Design review of the part built by this model. Coordinates are the model's own, in mm. A direction names the side the tool comes from. Give positions to 0.01 mm unless a question says otherwise; leave off trailing zeros. Loops run counter-clockwise (first coordinate to the right, second up) from the corner with the lowest first, then second, coordinate; pieces in that order, holes last. Notation, with made-up numbers: (-26, 86) - (28, 86) arc R24 cw to (28, 111) - close; hole circle Ø2 at (7, 18.25). An arc over 180 degrees is marked (long way). Put each result on its own line as item: value. Start each with the question number.
```python
from build123d import *

# Parameters (mm, degrees)
F1_DEPTH = 314.325
F2_R     = 3.175
F3_DEPTH = 50.801
F4_R     = 3.175
F5_DEPTH = 50.801


with BuildPart() as f1:
    # F0 (on Right) → F1 (new body, symmetric)
    with BuildSketch(Plane.YZ):
        Polygon((0, 44.45), (0, 0), (6.35, 0), (6.35, 50.8), (-44.45, 50.8), (-44.45, 44.45), align=None)
    extrude(amount=F1_DEPTH, both=True)

    # F2 (on face) → F3 (cut, through all)
    with BuildSketch(Plane.XY.offset(50.8)):
        with Locations((-298.45, -19.05)):
            Circle(F2_R)
        with Locations((-105.56875, -19.05)):
            Circle(F2_R)
        with Locations((298.45, -19.05)):
            Circle(F2_R)
        with Locations((-148.43125, -19.05)):
            Circle(F2_R)
        with Locations((-21.43125, -19.05)):
            Circle(F2_R)
        with Locations((21.43125, -19.05)):
            Circle(F2_R)
        with Locations((105.56875, -19.05)):
            Circle(F2_R)
        with Locations((148.43125, -19.05)):
            Circle(F2_R)
    extrude(amount=-F3_DEPTH, mode=Mode.SUBTRACT)

    # F4 (on face) → F5 (cut, through all)
    with BuildSketch(Plane.XY.offset(50.8)):
        with Locations((-185.166, -19.05)):
            Circle(F4_R)
        with Locations((-61.722, -19.05)):
            Circle(F4_R)
        with Locations((61.722, -19.05)):
            Circle(F4_R)
        with Locations((185.166, -19.05)):
            Circle(F4_R)
    extrude(amount=-F5_DEPTH, mode=Mode.SUBTRACT)


solid = f1.part
```
Item 1: Consider section B-B (x = -123). State the section outline as (y, z) points, plus the area to 3 significant figures.
Item 2: For L1, parallel to Y at x = 272, z = 24; L2, parallel to Z at x = 264, y = -40.5; L3, parallel to Y at x = 298.45, z = 47.25 (3 decimals), list the stretches that pass through material, from the lowest coordinate up. Write a range as from..to.
Item 3: Consider section A-A (y = -36.5). State the section outline as (x, z) points (3 decimals), plus the area to 3 significant figures.
Item 4: Consider section C-C (z = 29.5). State the section outline as (x, y) points (3 decimals).
Item 5: For P1, Ø5.5, axis at x = 148.43, y = -19.05, coming from the -Z side; P2, Ø7.5, axis at x = -21.43, y = -19.05, coming from the -Z side, all flat-tipped, find the tip position at first contact; note any pin that passes through.
Item 6: Machinability: for faces 1 (the flat face through (4, -19, 50.8)), 2 (the flat face through (4, 0, 23)), which of the approach directions +Z, -Z, +X, -X, +Y, -Y give a long, thin tool a straight path to every point of the face, cutting with its end or side? Answer none if there is none.
Geometry says:
1. outline: (-44.45, 44.45) - (0, 44.45) - (0, 0) - (6.35, 0) - (6.35, 50.8) - (-44.45, 50.8) - close
1. area: 605 mm2
2. L1: y = 0..6.35
2. L2: z = 44.45..50.8
2. L3: y = -44.45..-22.225, -15.875..6.35
3. outline: (-314.325, 44.45) - (314.325, 44.45) - (314.325, 50.8) - (-314.325, 50.8) - close
3. area: 3,990 mm2
4. outline: (-314.325, 0) - (314.325, 0) - (314.325, 6.35) - (-314.325, 6.35) - close
5. P1: passes through
5. P2: stops at z = 44.45
6. face 1: +Z, +X, -X, +Y, -Y
6. face 2: -Z, +X, -X, -Y
